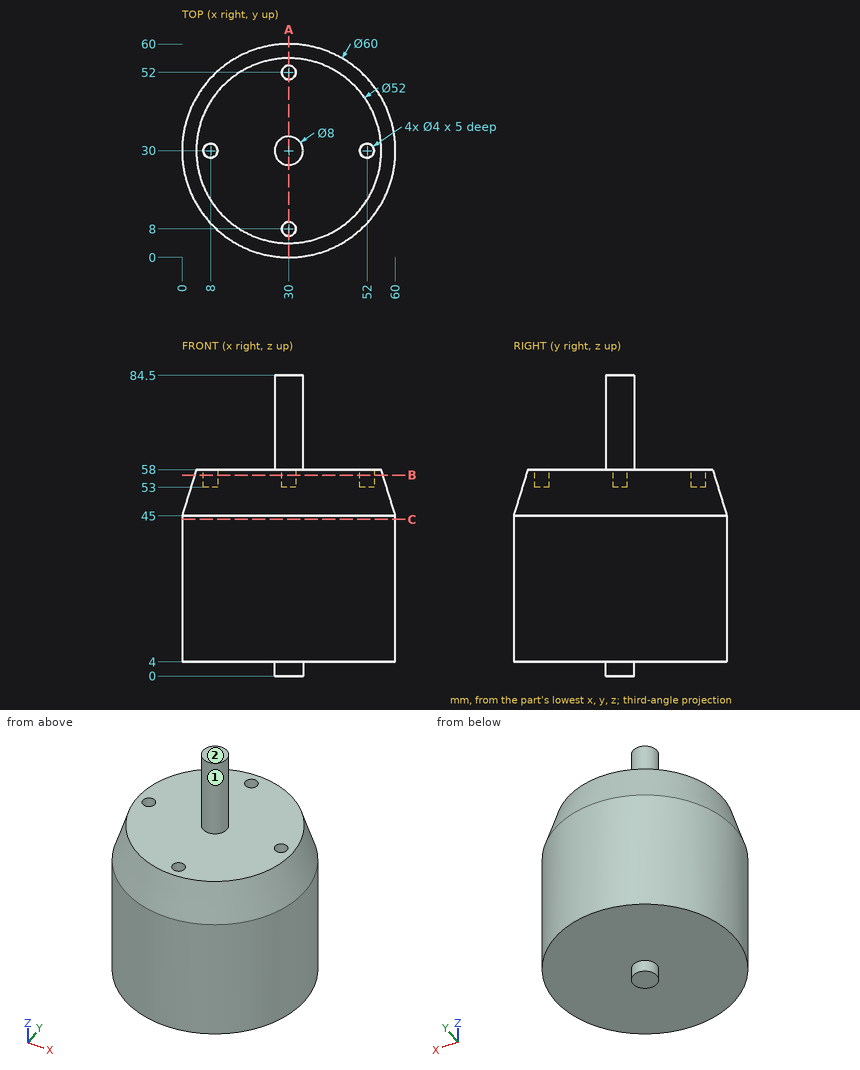
Part print with two shaded views. Sizes in mm from the minimum x, y, z corner. A direction names the side the tool comes from. Round coordinates to 2 decimals unless told otherwise and drop trailing zeros. Loops run counter-clockwise (first coordinate to the right, second up) from the corner with the lowest first, then second, coordinate; pieces in that order, holes last. Notation, with made-up numbers: (-13.75, 1) - (6.25, 1) arc R31 ccw to (6.25, 40) - close; hole circle Ø8 at (-18.5, 65). An arc over 180 degrees is marked (long way). Answer as a JSON object with one key per item and string values.
Item 1: Pin check, flat tips, straight feed: pin 1 (5 mm diameter, centred on x = 31.5, z = 54.5, fed in from +Y); pin 2 (3 mm diameter, centred on x = 29.5, y = 7, fed in from +Z); pin 3 (6.5 mm diameter, centred on x = 52, y = 30, fed in from -Z). Stop position of each tip, or through.
Output:
{"pin 1": "y = 57.81", "pin 2": "z = 58", "pin 3": "z = 4"}
Item 2: Band-saw the part on A-A on x = 30. List the corners of the cut face in (y, z), plus the area to 3 significant figures.
Output:
{"outline": "(0, 4) - (26, 4) - (26, 0) - (34, 0) - (34, 4) - (60, 4) - (60, 45) - (56, 58) - (54, 58) - (54, 53) - (50, 53) - (50, 58) - (34, 58) - (34, 84.5) - (26, 84.5) - (26, 58) - (10, 58) - (10, 53) - (6, 53) - (6, 58) - (4, 58) - (0, 45) - close", "area": "3,390 mm2"}
Item 3: Band-saw the part on C-C on z = 44. List the corners of the cut face in (x, y).
Output:
{"outline": "circle Ø60 at (30, 30)"}
Item 4: Band-saw the part on B-B on z = 56.5. List the corners of the cut face in (x, y).
Output:
{"outline": "circle Ø52.92 at (30, 30); hole circle Ø4 at (8, 30); hole circle Ø4 at (30, 8); hole circle Ø4 at (30, 52); hole circle Ø4 at (52, 30)"}
Item 5: Tool access for the marked faces 1 and 2: list every direction of +Z, -Z, +X, -X, +Y, -Y with a clear straight run to the whole face (end or side of a thin tool).
Output:
{"face 1": "+Z", "face 2": "+Z, +X, -X, +Y, -Y"}
Item 6: Wall check: L1, parallel to Y at x = 30, z = 54.6; L2, parallel to Z at x = 7.5, y = 25.5; L3, parallel to Y at x = 8, z = 55.7. Give the ranges that are in metal, low to high.
Output:
{"L1": "2.95 to 6, 10 to 50, 54 to 57.05", "L2": "4 to 58", "L3": "14.86 to 28, 32 to 45.14"}
